Input: part model. Units: mm. Frame: model coordinates. A direction names the side the tool comes from. Coordinates: 2 decimals unless noted, no trailing zeros. Loops run counter-clockwise (first coordinate to the right, second up) from the corner with the lowest first, then second, coordinate; pieces in that order, holes last.
(1) Section B-B, the plane y = 0. Return loops of the section in (x, z), then the cut area to 3 significant figures.
(2) Mould query, pull axis X, two halves, no side actions, for faces 1 (the face through (-3.83, -3, 5)), 2 (the face through (-3, -6, 8.5)), 3 (the face through (17.509, -5, 4)). Classes: released by +X, released by -X, zero draft, split by the parting line, or undercut.
(3) Section A-A, the plane y = -3.5. Return loops of the section in (x, z).
(4) Line query: L1, parallel to X at y = -3.25, z = 2; L2, parallel to X at y = 0, z = 6; L3, parallel to Y at x = 4.75, z = 1.25. Output: solid intervals per line, ascending.
(5) Section D-D, the plane y = 4.5. Return loops of the section in (x, z), then the cut area to 3 significant figures.
(6) Set-up query: faces 4 (the face through (13.105, -3, 5)), 5 (the face through (-4.129, 8.327, 5.07)), 6 (the face through (12, -6, 8.5)). Return all of +Z, -Z, +X, -X, +Y, -Y with unobstructed straight access to the full face (end or side cutting, diameter ignored); none if empty.
(7) Section C-C, the plane z = 6.75. Return loops of the section in (x, y), then the cut area to 3 significant figures.
(8) Contact query for flat-ended pins moving along their axis: P1, Ø4, axis at x = -7.5, z = 4.5, coming from the -Y side; P2, Ø0.8, axis at x = -2.5, z = 9, coming from the -Y side; P3, Ø4, axis at x = -5.5, z = 7.5, coming from the +Y side; P4, Ø0.8, axis at y = -0.5, z = 9.5, coming from the -X side. Output: stop coordinate, or through.
Autodesk Inventor part; units mm, degrees
ref_plane "YZ Plane" through (0, 0, 0) normal (1, 0, 0) x (0, 1, 0)
ref_plane "XZ Plane" through (0, 0, 0) normal (0, 1, 0) x (-1, 0, 0)
ref_plane "XY Plane" through (0, 0, 0) normal (0, 0, 1) x (1, 0, 0)
sketch "스케치1" plane through (0, 0, 0) normal (0, 0, 1) x (1, 0, 0)
  line L0 (0, 11.2555) -> (-9.6591, 11.2555)
  line L1 (-9.6591, 11.2555) -> (-9.6591, -14.4887)
  line L2 (-9.6591, -14.4887) -> (0, -14.4887)
  line L3 (0, -14.4887) -> (0, 11.2555)
  point P0 (0, 0)
extrude "돌출1" add sketch "스케치1" along normal blind 10
sketch "스케치2" plane through (0, 0, 10) normal (0, 0, 1) x (1, 0, 0)
  line L0 (0, 11.2555) -> (-9.6591, 11.2555)
  line L1 (0, -14.4887) -> (0, 11.2555)
  line L2 (-8.1436, 11.2555) -> (0, 5.3146)
  line L3 (0, 5.3146) -> (9.2752, 5.3146)
  line L4 (9.2752, 5.3146) -> (9.2752, -14.4887)
  line L5 (9.2752, -14.4887) -> (0, -14.4887)
  line L6 (0, -14.4887) -> (0, 5.3146)
  circle A0 centre (4.6376, 0) radius 2.0297
  circle A1 centre (4.6376, -10.4068) radius 1.7507
  line L7 (0, 2.0297) -> (-9.6591, 2.0297)
  line L8 (-9.6591, 2.0297) -> (-9.6591, -14.4887)
  line L9 (-9.6591, -14.4887) -> (0, -14.4887)
  line L10 (0, -14.4887) -> (0, 2.0297)
  arc A2 (-3.8296, 3.0291) -> (-5.8296, 3.0291) centre (-4.8296, 3.0291) ccw
  arc A3 (-5.8296, -9.1284) -> (-3.8296, -9.1284) centre (-4.8296, -9.1284) ccw
  line L11 (-5.8296, 3.0291) -> (-5.8296, -9.1284)
  line L12 (-3.8296, 3.0291) -> (-3.8296, -9.1284)
  point P0 (0, 0)
  dimension "d2" = 2
  dimension "d3" = 2
extrude "돌출2" add sketch "스케치2" against normal blind 10 contours L3 L4 L5 L1
extrude "돌출3" add sketch "스케치2" along normal blind 1.25 contours L3 L4 L5 L1
extrude "돌출4" cut sketch "스케치2" against normal up to next contours L1 L2 L0
extrude "돌출5" cut sketch "스케치2" against normal up to next contours L12 A3 L11 L7 | L7 L11 A2 L12
extrude "돌출6" cut sketch "스케치2" against normal blind 1.5 contours L1 L9 L8 L7 L11 A3 L12 | L12 A3 L11 L7
sketch "스케치3" plane through (0, 0, 8.5) normal (0, 0, 1) x (1, 0, 0)
  line L0 (0, -14.4887) -> (-9.6591, -14.4887)
  line L1 (-9.6591, 2.0297) -> (-8.1436, 2.0297)
  line L2 (-8.1436, 2.0297) -> (-8.1436, -14.4887)
  line L3 (-8.1436, -14.4887) -> (-9.6591, -14.4887)
  line L4 (-9.6591, -14.4887) -> (-9.6591, 2.0297)
  point P0 (0, 0)
extrude "돌출7" cut sketch "스케치3" against normal up to next
chamfer "모따기1" distance 2 angle 45 1 edges at (-8.1436, -14.4887, 4.25)
sketch "스케치4" plane through (0, 0, 11.25) normal (0, 0, 1) x (1, 0, 0)
  line L0 (0, -14.4887) -> (9.2752, -14.4887)
  line L1 (9.2752, 5.3146) -> (4.6376, 5.3146)
  line L2 (4.6376, 5.3146) -> (4.6376, -14.4887)
  line L3 (4.6376, -14.4887) -> (9.2752, -14.4887)
  line L4 (9.2752, -14.4887) -> (9.2752, 5.3146)
  point P0 (0, 0)
extrude "돌출8" cut sketch "스케치4" against normal up to next
mirror "대칭1" about plane through (4.6376, -14.4887, 11.25) normal (1, 0, 0) of "돌출4", "돌출2", "돌출3", "돌출1", "돌출6", "돌출5"
sketch "스케치5" plane through (9.2752, -14.4887, 8.5) normal (0, 0, 1) x (1, 0, 0)
  line L0 (9.6591, 0) -> (0, 0)
  line L1 (9.6591, 16.5185) -> (8.2337, 16.5185)
  line L2 (8.2337, 16.5185) -> (8.2337, 0)
  line L3 (8.2337, 0) -> (9.6591, 0)
  line L4 (9.6591, 0) -> (9.6591, 16.5185)
  point P0 (-9.2752, 14.4887)
extrude "돌출9" cut sketch "스케치5" against normal up to next
chamfer "모따기2" distance 2 angle 45 1 edges at (17.5089, -14.4887, 4.25)
properties part number "240710_part1"
Report:
1. outline: (-8.14, 0) - (-5.83, 0) - (-5.83, 8.5) - (-8.14, 8.5) - close; (-3.83, 0) - (2.61, 0) - (2.61, 11.25) - (0, 11.25) - (0, 8.5) - (-3.83, 8.5) - close; (6.67, 0) - (13.1, 0) - (13.1, 8.5) - (9.28, 8.5) - (9.28, 11.25) - (6.67, 11.25) - close; (15.1, 0) - (17.51, 0) - (17.51, 8.5) - (15.1, 8.5) - close
1. area: 164 mm2
2. face 1: undercut
2. face 2: zero draft
2. face 3: released by +X
3. outline: (-8.14, 0) - (-5.83, 0) - (-5.83, 8.5) - (-8.14, 8.5) - close; (-3.83, 0) - (13.1, 0) - (13.1, 8.5) - (9.28, 8.5) - (9.28, 11.25) - (0, 11.25) - (0, 8.5) - (-3.83, 8.5) - close; (15.1, 0) - (17.51, 0) - (17.51, 8.5) - (15.1, 8.5) - close
4. L1: x = -8.14 to -5.83, -3.83 to 13.1, 15.1 to 17.51
4. L2: x = -8.14 to -5.83, -3.83 to 2.61, 6.67 to 13.1, 15.1 to 17.51
4. L3: y = -14.49 to -12.15, -8.66 to -2.03, 2.03 to 5.31
5. outline: (-9.66, 0) - (18.93, 0) - (18.93, 10) - (9.28, 10) - (9.28, 11.25) - (0, 11.25) - (0, 10) - (-9.66, 10) - close
5. area: 298 mm2
6. face 4: +Z, -Z
6. face 5: +Z, -Z, +Y
6. face 6: +Z, +X, -Y
7. outline: (-9.66, 2.03) - (-8.14, 2.03) - (-8.14, -12.49) - (-6.14, -14.49) - (15.51, -14.49) - (17.51, -12.49) - (17.51, 2.03) - (18.93, 2.03) - (18.93, 11.26) - (17.42, 11.26) - (9.28, 5.31) - (0, 5.31) - (-8.14, 11.26) - (-9.66, 11.26) - close; hole (-5.83, -9.13) arc R1 ccw to (-3.83, -9.13) - (-3.83, 3.03) arc R1 ccw to (-5.83, 3.03) - close; hole circle Ø4.06 at (4.64, 0); hole circle Ø3.5 at (4.64, -10.41); hole (13.1, -9.13) arc R1 ccw to (15.1, -9.13) - (15.1, 3.03) arc R1 ccw to (13.1, 3.03) - close
7. area: 503 mm2
8. P1: stops at y = -14.49
8. P2: stops at y = 2.03
8. P3: stops at y = 10.79
8. P4: stops at x = 0
